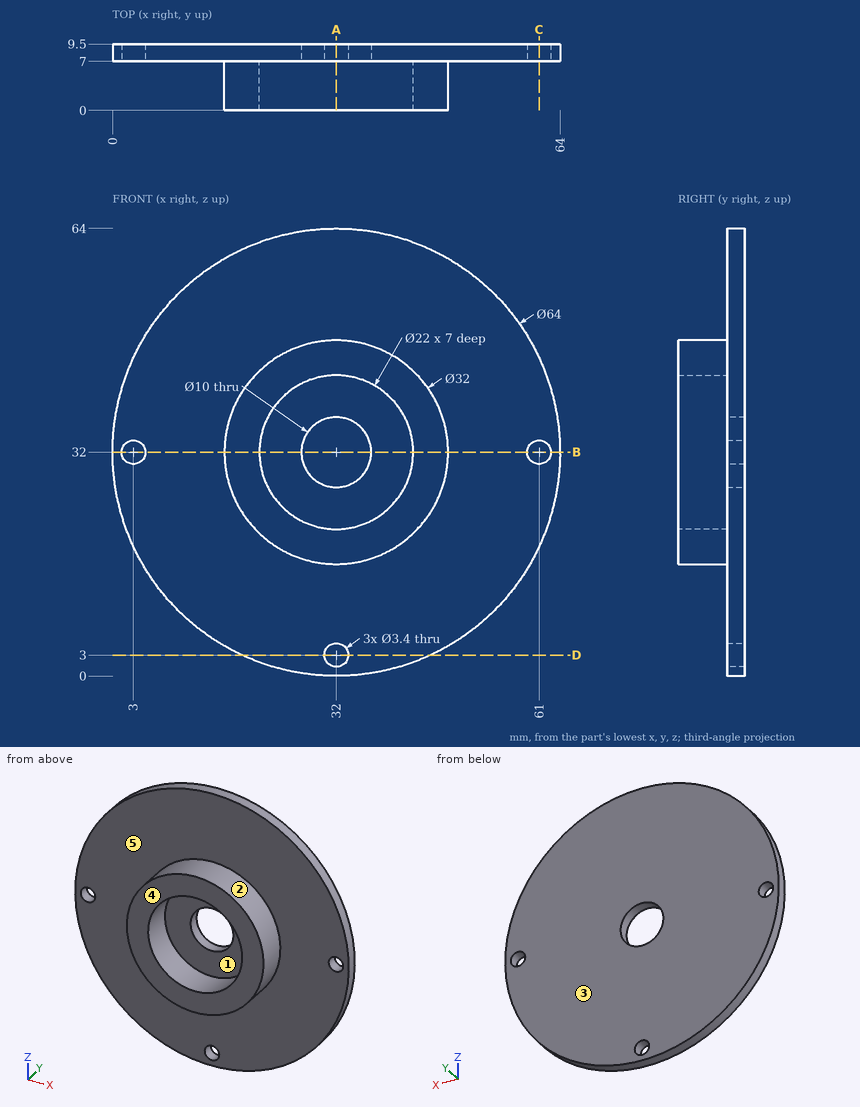
Part print with two shaded views. Sizes in mm from the minimum x, y, z corner. A direction names the side the tool comes from. Round coordinates to 2 decimals unless told otherwise and drop trailing zeros. Loops run counter-clockwise (first coordinate to the right, second up) from the corner with the lowest first, then second, coordinate; pieces in that order, holes last. Notation, with made-up numbers: (-16, 18) - (21, 18) arc R19 ccw to (21, 53) - close; hole circle Ø11 at (41, 74.25). An arc over 180 degrees is marked (long way). Answer as a JSON object with one key per item and string values.
Item 1: Band-saw the part on D-D on z = 3. List the corners of the cut face in (x, y), plus the area to 3 significant figures.
Output:
{"outline": "(18.47, 7) - (30.3, 7) - (30.3, 9.5) - (18.47, 9.5) - close; (33.7, 7) - (45.53, 7) - (45.53, 9.5) - (33.7, 9.5) - close", "area": "59.1 mm2"}
Item 2: Wall check: L1, parallel to X at y = 7.9, z = 32; L2, parallel to X at y = 2.75, z = 32; L3, parallel to Y at x = 58, z = 45. Give the ranges that are in metal, low to high.
Output:
{"L1": "0 to 1.3, 4.7 to 27, 37 to 59.3, 62.7 to 64", "L2": "16 to 21, 43 to 48", "L3": "7 to 9.5"}
Item 3: Tool access for the marked faces 4 and 5: list every direction of +Z, -Z, +X, -X, +Y, -Y with a clear straight run to the whole face (end or side of a thin tool).
Output:
{"face 4": "+Z, -Z, +X, -X, -Y", "face 5": "-Y"}
Item 4: Band-saw the part on C-C on x = 61. List the corners of the cut face in (y, z), plus the area to 3 significant figures.
Output:
{"outline": "(7, 18.47) - (9.5, 18.47) - (9.5, 30.3) - (7, 30.3) - close; (7, 33.7) - (9.5, 33.7) - (9.5, 45.53) - (7, 45.53) - close", "area": "59.1 mm2"}
Item 5: Pull direction X, two halves, no side cores. Call the marked faces 1, 2 and 3: pulls with the +X half, pulls with the -X half, needs draft (parallel to the pull), parting line crosses it, or undercut.
Output:
{"face 1": "undercut", "face 2": "parting line crosses it", "face 3": "needs draft"}
Item 6: Band-saw the part on B-B on z = 32. List the corners of the cut face in (x, y), plus the area to 3 significant figures.
Output:
{"outline": "(0, 7) - (1.3, 7) - (1.3, 9.5) - (0, 9.5) - close; (4.7, 7) - (16, 7) - (16, 0) - (21, 0) - (21, 7) - (27, 7) - (27, 9.5) - (4.7, 9.5) - close; (37, 7) - (43, 7) - (43, 0) - (48, 0) - (48, 7) - (59.3, 7) - (59.3, 9.5) - (37, 9.5) - close; (62.7, 7) - (64, 7) - (64, 9.5) - (62.7, 9.5) - close", "area": "188 mm2"}
Item 7: Pin check, flat tips, straight feed: pin 1 (1.5 mm diameter, centred on y = 7.5, z = 9, fed in from +X); pin 2 (8 mm diameter, centred on x = 32, z = 32, fed in from -Y); pin 3 (4 mm diameter, centred on x = 8.5, y = 5.5, fed in from -Z); pin 4 (5.5 mm diameter, centred on x = 3, z = 32, fed in from -Y). Stop position of each tip, or through.
Output:
{"pin 1": "x = 55", "pin 2": "through", "pin 3": "z = 8.93", "pin 4": "y = 7"}
Item 8: Band-saw the part on A-A on x = 32. List the corners of the cut face in (y, z), plus the area to 4 significant figures.
Output:
{"outline": "(0, 16) - (7, 16) - (7, 4.7) - (9.5, 4.7) - (9.5, 27) - (7, 27) - (7, 21) - (0, 21) - close; (0, 43) - (7, 43) - (7, 37) - (9.5, 37) - (9.5, 64) - (7, 64) - (7, 48) - (0, 48) - close; (7, 0) - (9.5, 0) - (9.5, 1.3) - (7, 1.3) - close", "area": "196.5 mm2"}
